Autodesk Inventor part; units mm, degrees
ref_plane "YZ Plane" through (0, 0, 0) normal (1, 0, 0) x (0, 1, 0)
ref_plane "XZ Plane" through (0, 0, 0) normal (0, 1, 0) x (-1, 0, 0)
ref_plane "XY Plane" through (0, 0, 0) normal (0, 0, 1) x (1, 0, 0)
sketch "Sketch1" plane through (0, 0, 0) normal (0, 0, 1) x (1, 0, 0)
  line L0 (25, 0) -> (25, 4)
  line L1 (0, 4) -> (25, 4)
  line L2 (0, 0) -> (0, 4)
  line L3 (16.65, -10.896) -> (12.5, -13.292)
  line L4 (12.5, -13.292) -> (8.35, -10.896)
  line L5 (8.35, -10.896) -> (8.35, -6.104)
  line L6 (16.65, -6.104) -> (16.65, -10.896)
  line L7 (8.35, -6.104) -> (8.35, 0)
  line L8 (16.65, -6.104) -> (16.65, 0)
  line L9 (25, -8.5) -> (25, 0)
  line L10 (0, -8.5) -> (0, 0)
  arc A0 (0, -8.5) -> (25, -8.5) centre (12.5, -8.5) ccw
  line L11 (10, -4.5) -> (10, -8.5)
  line L12 (15, -8.5) -> (15, -4.5)
  arc A1 (15, -4.5) -> (10, -4.5) centre (12.5, -4.5) ccw
  arc A2 (10, -8.5) -> (15, -8.5) centre (12.5, -8.5) ccw
  line L13 (-2, 0) -> (-2, -8.5)
  arc A3 (-2, -8.5) -> (27, -8.5) centre (12.5, -8.5) ccw
  line L14 (27, -8.5) -> (27, 0)
  line L15 (0, 0) -> (-2, 0)
  line L16 (-2, 0) -> (-5.3, 0)
  line L17 (-2, -4) -> (-12, -4)
  line L18 (-12, -4) -> (-12, 0)
  line L19 (-12, 0) -> (-8.7, 0)
  line L20 (27, -4) -> (37, -4)
  line L21 (37, -4) -> (37, 0)
  line L22 (37, 0) -> (33.7, 0)
  line L23 (25, 0) -> (27, 0)
  line L24 (27, 0) -> (30.3, 0)
  line L25 (25, 0) -> (16.65, 0)
  line L26 (8.35, 0) -> (16.65, 0)
  line L27 (8.35, 0) -> (0, 0)
  line L28 (33.7, 0) -> (30.3, 0)
  line L29 (-5.3, 0) -> (-8.7, 0)
  line L30 (32, 0) -> (32, -6.5) construction
  line L31 (-7, 0) -> (-7, -7.118) construction
  dimension "d5" = 8.3
  dimension "d7" = 5
  dimension "d8" = 2
  dimension "d9" = 4
  dimension "d10" = 4
  dimension "d13" = 8.5
  dimension "d14" = 12.5
extrude "Extrusion1" add sketch "Sketch1" along normal blind 12 contours L23 L14 A3 L13 L15 L10 A0 L9 | L24 L28 L22 L21 L20 L14 | L13 L17 L18 L19 L29 L16
sketch "Sketch2" plane through (0, 0, 0) normal (0, 0, -1) x (-1, 0, 0)
  line L0 (-25, 0) -> (-25, -8.5)
  arc A0 (-25, -8.5) -> (0, -8.5) centre (-12.5, -8.5) ccw
  line L1 (0, -8.5) -> (0, 0)
  line L2 (-27, -8.5) -> (-27, 0)
  arc A1 (-27, -8.5) -> (2, -8.5) centre (-12.5, -8.5) ccw
  line L3 (2, 0) -> (2, -8.5)
  line L4 (-8.35, -6.104) -> (-8.35, 0)
  line L5 (-8.35, -10.896) -> (-8.35, -6.104)
  line L6 (-12.5, -13.292) -> (-8.35, -10.896)
  line L7 (-16.65, -10.896) -> (-12.5, -13.292)
  line L8 (-16.65, -6.104) -> (-16.65, -10.896)
  line L9 (-16.65, -6.104) -> (-16.65, 0)
  line L10 (-15, -8.5) -> (-15, -4.5)
  arc A2 (-10, -4.5) -> (-15, -4.5) centre (-12.5, -4.5) ccw
  line L11 (-10, -4.5) -> (-10, -8.5)
  arc A3 (-15, -8.5) -> (-10, -8.5) centre (-12.5, -8.5) ccw
  line L12 (-245.5, 0) -> (14.5, 0)
extrude "Extrusion2" add sketch "Sketch2" along normal blind 4 contours L12 L9 L8 L7 L6 L5 L4 L1 A0 L0 | L0 A0 L1 L12 L3 A1 L2
sketch "Sketch3" plane through (0, 0, 0) normal (0, 0, 1) x (1, 0, 0)
  line L0 (8.35, 0) -> (8.35, -10.896)
  line L1 (12.5, -13.292) -> (8.35, -10.896)
  line L2 (12.5, -13.292) -> (16.65, -10.896)
  line L3 (16.65, -10.896) -> (16.65, 0)
  line L4 (15, -8.5) -> (15, -4.5)
  arc A0 (10, -8.5) -> (15, -8.5) centre (12.5, -8.5) ccw
  line L5 (10, -4.5) -> (10, -8.5)
  arc A1 (15, -4.5) -> (10, -4.5) centre (12.5, -4.5) ccw
  line L6 (92, 0) -> (245.5, 0)
  line L7 (245.5, 0) -> (-14.5, 0)
  point P0 (0, 0)
extrude "Extrusion3" add sketch "Sketch3" against normal blind 2
sketch "Sketch4" plane through (0, 0, 12) normal (0, 0, 1) x (1, 0, 0)
  arc A0 (15, -4.5) -> (10, -4.5) centre (12.5, -4.5) ccw
  line L0 (10, -8.5) -> (10, -4.5)
  arc A1 (10, -8.5) -> (15, -8.5) centre (12.5, -8.5) ccw
  line L1 (15, -4.5) -> (15, -8.5)
  line L2 (25, 0) -> (25, -8.5)
  arc A2 (0, -8.5) -> (25, -8.5) centre (12.5, -8.5) ccw
  line L3 (0, -8.5) -> (0, 0)
  line L4 (0, 0) -> (-12, 0)
  line L5 (-12, 0) -> (-12, -4)
  line L6 (-12, -4) -> (-2, -4)
  line L7 (-2, -4) -> (-2, -8.5)
  arc A3 (-2, -8.5) -> (27, -8.5) centre (12.5, -8.5) ccw
  line L8 (27, -8.5) -> (27, -4)
  line L9 (27, -4) -> (37, -4)
  line L10 (37, -4) -> (37, 0)
  line L11 (37, 0) -> (25, 0)
  line L12 (25, 0) -> (0, 0)
  line L13 (-2, -8.5) -> (-2, -4)
  line L14 (-2, -4) -> (-2, 0)
  line L15 (27, 0) -> (27, -8.5)
  line L16 (27, -4) -> (27, 0)
extrude "Extrusion4" add sketch "Sketch4" along normal blind 2
fillet "Fillet1" radius 2 6 edges at (27, -6.25, 14) (-2, -6.25, 14) (12.5, -23, 14) (-2, -4.25, -4) (27, -4.25, -4) (12.5, -23, -4)
sketch "Sketch5" plane through (27, -4, 0) normal (0, -1, 0) x (1, 0, 0)
  line L0 (7.85, 7.6454) -> (7.85, 4.3546)
  line L1 (7.85, 4.3546) -> (5, 2.7091)
  line L2 (5, 2.7091) -> (2.15, 4.3546)
  line L3 (2.15, 4.3546) -> (2.15, 7.6454)
  line L4 (2.15, 7.6454) -> (5, 9.2909)
  line L5 (5, 9.2909) -> (7.85, 7.6454)
  line L6 (-31.15, 7.6454) -> (-31.15, 4.3546)
  line L7 (-31.15, 4.3546) -> (-34, 2.7091)
  line L8 (-34, 2.7091) -> (-36.85, 4.3546)
  line L9 (-36.85, 4.3546) -> (-36.85, 7.6454)
  line L10 (-36.85, 7.6454) -> (-34, 9.2909)
  line L11 (-34, 9.2909) -> (-31.15, 7.6454)
  line L12 (10, 0) -> (10, 14)
  line L13 (-39, 0) -> (-39, 14)
  circle A0 centre (5, 6) radius 1.7
  circle A1 centre (-34, 6) radius 1.7
  point P0 (-27, 0)
  point P1 (10, 12)
  point P2 (-39, 12)
  dimension "d22" = 5.7
  dimension "d23" = 5.7
extrude "Extrusion5" cut sketch "Sketch5" against normal blind 2 contours L0 L1 L2 L3 L4 L5 | L6 L7 L8 L9 L10 L11 | A0 | A1
hole "Hole1" at (32, -4, 6) at (-7, -4, 6) direction (0, 1, 0) diameter 3.4 end through all
properties part number "bearing_holder"
CAD build for the part. Positions are in the model's coordinates, mm. A direction names the side the tool comes from. Round coordinates to 2 decimals unless told otherwise and drop trailing zeros. Loops run counter-clockwise (first coordinate to the right, second up) from the corner with the lowest first, then second, coordinate; pieces in that order, holes last. Notation, with made-up numbers: (-38, -7) - (20, -7) arc R22 cw to (20, 4) - close; hole circle Ø2 at (-36.5, 80). An arc over 180 degrees is marked (long way). Return JSON: item names as keys, results as strings. Group by question number.
Q1. Band-saw the part on B-B on z = 6. Give the cut face in (x, y), plus the area to 3 significant figures.
Q2. Flat gauge pins, fed straight in: pin 1 Ø4.5 at (x, y) = (30.5, -1.5) entering from -Z; pin 2 Ø1.5 at (x, z) = (9, 5) entering from -Y; pin 3 Ø1.5 at (x, z) = (28.5, 4) entering from -Y. Where does each tip first touch, or does it go through?
Q3. Band-saw the part on C-C on z = 10.25. Give the cut face in (x, y), plus the area to 3 significant figures.
Q4. Drill centre lines: line 1 along X through (y, z) = (-0.65, 6); line 2 along Z through (x, y) = (19, -11); line 3 along Z through (x, y) = (-7, -0.75). Where is each one in solid material? Low to high. Write a range as [from, to].
Q5. Band-saw the part on A-A on x = 31. Give the cut face in (y, z).
Q6. Two-plate mould, pull along Z, no slides. Class faces 1 (the face through (-5.56, -3.01, 3.54)), 2 (the face through (14.6, -12.08, -2.99)), 3 (the face through (9.7, -5.1, -2)): +Z half, -Z half, draft (parallel to the pull), parting line (faces both ways), or undercut.
Q7. Tool access for faces 4 (the face through (15, -10, 0)), 5 (the face through (34.85, -3, 6)), 6 (the face through (10.45, -12.11, -2.99)): list every direction of +Z, -Z, +X, -X, +Y, -Y with a clear straight run to the whole face (end or side of a thin tool).
Solutions:
{
 "1": {"outline": "(-12, -4) - (-9.85, -4) - (-9.85, -2) - (-8.7, -2) - (-8.7, 0) - (-12, 0) - close; (-5.3, -2) - (-4.15, -2) - (-4.15, -4) - (-2, -4) - (-2, -8.5) arc R14.5 ccw to (27, -8.5) - (27, -4) - (29.15, -4) - (29.15, -2) - (30.3, -2) - (30.3, 0) - (25, 0) - (25, -8.5) arc R12.5 cw to (0, -8.5) - (0, 0) - (-5.3, 0) - close; (33.7, -2) - (34.85, -2) - (34.85, -4) - (37, -4) - (37, 0) - (33.7, 0) - close", "area": "162 mm^2"},
 "2": {"pin 1": "stops at z = 0", "pin 2": "stops at y = -22.74", "pin 3": "stops at y = -4"},
 "3": {"outline": "(-12, -4) - (-2, -4) - (-2, -8.5) arc R14.5 ccw to (27, -8.5) - (27, -4) - (37, -4) - (37, 0) - (25, 0) - (25, -8.5) arc R12.5 cw to (0, -8.5) - (0, 0) - (-12, 0) - close", "area": "199 mm^2"},
 "4": {"line 1": "x = [-12, -8.7], [-5.3, 0], [25, 30.3], [33.7, 37]", "line 2": "z = [-4, 0], [12, 14]", "line 3": "z = [0, 4.3], [7.7, 14]"},
 "5": {"outline": "(-4, 0) - (0, 0) - (0, 4.63) - (-2, 4.63) - (-2, 3.29) - (-4, 3.29) - close; (-4, 8.71) - (-2, 8.71) - (-2, 7.37) - (0, 7.37) - (0, 14) - (-4, 14) - close"},
 "6": {"face 1": "undercut", "face 2": "draft", "face 3": "-Z half"},
 "7": {"face 4": "+Y", "face 5": "-Y", "face 6": "-Z, +Y"}
}
